from build123d import *

# Parameters (mm, degrees)
ESQUISSE1_W             = 25
ESQUISSE1_H             = 18
ESQUISSE1_R             = 6
BOSS_EXTRU_1_DEPTH      = 5
ESQUISSE2_R             = 1
ENL_V_MAT_EXTRU_1_DEPTH = 15


with BuildPart() as part:
    # Esquisse1 → Boss.-Extru.1 (new body)
    with BuildSketch(Plane.XY):
        Rectangle(ESQUISSE1_W, ESQUISSE1_H)
        Circle(ESQUISSE1_R, mode=Mode.SUBTRACT)
    extrude(amount=BOSS_EXTRU_1_DEPTH)

    # Esquisse2 → Enlèv. mat.-Extru.1 (cut)
    with BuildSketch(Plane(origin=(0, 9, 0), x_dir=(1, 0, 0), z_dir=(0, 1, 0))):
        with Locations((-8, -2.5)):
            Circle(ESQUISSE2_R)
        with Locations((8, -2.5)):
            Circle(ESQUISSE2_R)
    extrude(amount=-ENL_V_MAT_EXTRU_1_DEPTH, mode=Mode.SUBTRACT)


solid = part.part
Geometry: final body of the model. Coordinates: model frame, mm. A direction names the side the tool comes from. Coordinates: 2 decimals unless noted, no trailing zeros. Order: outer loops, then holes, each group sorted by start corner. A loop starts at its lowest first (then second) coordinate and runs counter-clockwise, first axis right, second up.
(1) Material intervals for probe 1 along X at (y, z) = (5.5, 2.15); probe 2 along X at (y, z) = (-2.25, 2.5); probe 3 along Y at (x, z) = (0, 1.15), sorted ascending.
(2) Section query B-B (z = 2.5). Return the cut outline in (x, y).
(3) Section query C-C (y = -3.5). Return the cut outline in (x, z), plus the area to 3 significant figures.
(4) Draft query along X for faces 1 (the face through (-6, 2, 0)), 2 (the face through (-8, -6, 2)), 3 (the face through (-12.5, 0, 2)). Return one class per face: pulls with the +X half, pulls with the -X half, needs draft (parallel to the pull), parting line crosses it, or undercut.
(5) Access query for faces 4 (the face through (0, 9, 2)), 5 (the face through (-8.8, 1.6, 3.1)). Directions: +Z, -Z, +X, -X, +Y, -Y. A direction counts if a zero-diameter tool reaches every point of the face in a straight line with its end or side. Return the directions, or none.
(6) First-contact query: pin 1 (2 mm diameter, centred on x = 8, z = 2, fed in from +Y); pin 2 (1.2 mm diameter, centred on x = -8, z = 2.5, fed in from +Y). Flat tips, straight axial feed; report the tip coordinate or a pass-through.
(7) Section query A-A (x = 0). Return the cut outline in (y, z).
(8) Section query D-D (x = -8). Return the cut outline in (y, z).
Solution:
1. probe 1: x = -12.5 to -8.94, -7.06 to -2.4, 2.4 to 7.06, 8.94 to 12.5
1. probe 2: x = -12.5 to -9, -7 to -5.56, 5.56 to 7, 9 to 12.5
1. probe 3: y = -9 to -6, 6 to 9
2. outline: (-12.5, -9) - (12.5, -9) - (12.5, 9) - (9, 9) - (9, -6) - (7, -6) - (7, 9) - (-7, 9) - (-7, -6) - (-9, -6) - (-9, 9) - (-12.5, 9) - close; hole circle Ø12 at (0, 0)
3. outline: (-12.5, 0) - (-4.87, 0) - (-4.87, 5) - (-12.5, 5) - close; (4.87, 0) - (12.5, 0) - (12.5, 5) - (4.87, 5) - close; hole circle Ø2 at (-8, 2.5); hole circle Ø2 at (8, 2.5)
3. area: 70.0 mm2
4. face 1: needs draft
4. face 2: undercut
4. face 3: pulls with the -X half
5. face 4: +Z, -Z, +X, -X, +Y
5. face 5: +Y
6. pin 1: stops at y = 9
6. pin 2: stops at y = -6
7. outline: (-9, 0) - (-6, 0) - (-6, 5) - (-9, 5) - close; (6, 0) - (9, 0) - (9, 5) - (6, 5) - close
8. outline: (-9, 0) - (9, 0) - (9, 1.5) - (-6, 1.5) - (-6, 3.5) - (9, 3.5) - (9, 5) - (-9, 5) - close
